```python
from build123d import *

# Parameters (mm, degrees)
F0_W      = 167.5
F0_H      = 92
F1_DEPTH  = 5.5
F2_W      = 137.5
F2_H      = 92
F3_DEPTH  = 49.7
F4_R      = 10
F5_R      = 2.54
F6_R      = 3.3
F6_R_2    = 3
F7_DEPTH  = 5.5
F10_DEPTH = 5.5
F11_R     = 5
F12_R     = 11.129920483
F12_R_2   = 9.5443004054
F13_DEPTH = 10


# Not quite as in the source:
# - a feature names something its author has since deleted; it is built from what else it names


with BuildPart() as f1:
    # F0 (on Top) → F1 (new body)
    with BuildSketch(Plane.XY):
        Rectangle(F0_W, F0_H)
    extrude(amount=F1_DEPTH)

    # F2 (on Top) → F3 (join)
    with BuildSketch(Plane.XY):
        Rectangle(F2_W, F2_H)
    extrude(amount=F3_DEPTH)

    # F4
    f4_edges = [f1.edges().sort_by_distance(p)[0] for p in [
        (-83.75, -46, 2.75),
        (83.75, -46, 2.75),
        (83.75, 46, 2.75),
        (-83.75, 46, 2.75),
        (-68.75, 46, 27.6),
        (-68.75, -46, 27.6),
        (68.75, 46, 27.6),
        (68.75, -46, 27.6),
    ]]
    fillet(f4_edges, radius=F4_R)

    # F5
    f5_edges = [f1.edges().sort_by_distance(p)[0] for p in [
        (0, -46, 49.7),
        (0, 46, 49.7),
        (65.821068, -43.071068, 49.7),
        (68.75, 0, 49.7),
        (65.821068, 43.071068, 49.7),
        (-65.821068, -43.071068, 49.7),
        (-68.75, 0, 49.7),
        (-65.821068, 43.071068, 49.7),
    ]]
    fillet(f5_edges, radius=F5_R)

    # F6 (on face) → F7 (cut)
    with BuildSketch(Plane.XY.offset(5.5)):
        with Locations((-76.25, 22.5)):
            Circle(F6_R)
        with Locations((-76.25, -22.5)):
            Circle(F6_R)
        with Locations((76.25, -22.5)):
            Circle(F6_R)
        with Locations((76.25, 22.5)):
            Circle(F6_R)
        with Locations((76.25, 37.4)):
            Circle(F6_R_2)
        with Locations((76.25, -37.4)):
            Circle(F6_R_2)
    extrude(amount=-F7_DEPTH, mode=Mode.SUBTRACT)

    # F8 (on face) + F9 (on face) → F10 (cut)
    with BuildSketch(Plane.XY.offset(5.5)):
        with BuildLine():
            ThreePointArc((-83.75, -15), (-73.1433982822, -10.6066017178), (-68.75, 0))
            ThreePointArc((-68.75, 0), (-73.1433982822, 10.6066017178), (-83.75, 15))
            Line((-83.75, 15), (-83.75, -15))
        make_face()
    with BuildSketch(Plane.XY.offset(5.5)):
        with BuildLine():
            Line((83.75, -15), (83.75, 15))
            ThreePointArc((83.75, 15), (73.1433983426, 10.6066017782), (68.75, 1.709e-07))
            ThreePointArc((68.75, 1.709e-07), (73.1433982218, -10.6066016574), (83.75, -15))
        make_face()
    extrude(amount=-F10_DEPTH, mode=Mode.SUBTRACT)

    # F11
    f11_edges = [f1.edges().sort_by_distance(p)[0] for p in [
        (83.75, -15, 2.75),
        (-83.75, -15, 2.75),
        (-83.75, 15, 2.75),
        (83.75, 15, 2.75),
    ]]
    fillet(f11_edges, radius=F11_R)

    # F12 (on face) → F13 (join)
    with BuildSketch(Plane.XY.offset(49.7)):
        with Locations((50.4262000322, -21.045640111)):
            Circle(F12_R)
        with Locations((46.4671105146, 16.4614468813)):
            Circle(F12_R_2)
    extrude(amount=F13_DEPTH)


solid = f1.part
```
Geometry check sheet. Reference: the model listing, model coordinates, mm. A direction names the side the tool comes from. Coordinates: 2 decimals unless noted, no trailing zeros. Order: outer loops, then holes, each group sorted by start corner. A loop starts at its lowest first (then second) coordinate and runs counter-clockwise, first axis right, second up. Notation, with made-up numbers: M 48,-32.5 L 94,-32.5 A25 cw 94,2.5 Z; hole C -3,23 d8. An arc over 180 degrees is marked long. Answer as a JSON object with one key per item and string values.
Q1. Cross-section at A-A on x = -76.25. Record the cut outline in (y, z), and give its area (3 significant figures).
Results are:
{"outline": "M -45.68,0 L -25.8,0 L -25.8,5.5 L -45.68,5.5 Z; M -19.2,0 L -12.99,0 L -12.99,5.5 L -19.2,5.5 Z; M 12.99,0 L 19.2,0 L 19.2,5.5 L 12.99,5.5 Z; M 25.8,0 L 45.68,0 L 45.68,5.5 L 25.8,5.5 Z", "area": "287 mm²"}
Q2. Cross-section at B-B on z = 20.5. Record the cut outline in (x, y), and give its area (3 significant figures).
Results are:
{"outline": "M -68.75,-36 A10 ccw -58.75,-46 L 58.75,-46 A10 ccw 68.75,-36 L 68.75,36 A10 ccw 58.75,46 L -58.75,46 A10 ccw -68.75,36 Z", "area": "12,600 mm²"}
Q3. Tool access check on faces 4 (the cylindrical face through (-82.7, 16.3, 2.7)), 5 (the cylindrical face through (82.7, 16.3, 2.7)), 6 (the cylindrical face through (55.6, -30.9, 54.6)), 7 (the cylindrical face through (65.74, 43.15, 26.62)). Record the directions out of +Z, -Z, +X, -X, +Y, -Y that give a thin tool (end or side, any length) a straight path to the whole face; none if there is none.
Results are:
{"face 4": "+Z, -Z, -X", "face 5": "+Z, -Z, +X", "face 6": "+Z", "face 7": "+Z, +X, +Y"}
Q4. Scan lines: line 1 (Y direction, x = 76, z = 1); line 2 (Y direction, x = -76, z = 1); line 3 (Z direction, x = -45.5, y = -13). Record each from-to range of solid material in increasing order.
Results are:
{"line 1": "y = -45.74 to -40.39, -34.41 to -25.79, -19.21 to -12.84, 12.84 to 19.21, 25.79 to 34.41, 40.39 to 45.74", "line 2": "y = -45.74 to -25.79, -19.21 to -12.84, 12.84 to 19.21, 25.79 to 45.74", "line 3": "z = 0 to 49.7"}
Q5. Cross-section at D-D on x = 76.25. Record the cut outline in (y, z).
Results are:
{"outline": "M -45.68,0 L -40.4,0 L -40.4,5.5 L -45.68,5.5 Z; M -34.4,0 L -25.8,0 L -25.8,5.5 L -34.4,5.5 Z; M -19.2,0 L -12.99,0 L -12.99,5.5 L -19.2,5.5 Z; M 12.99,0 L 19.2,0 L 19.2,5.5 L 12.99,5.5 Z; M 25.8,0 L 34.4,0 L 34.4,5.5 L 25.8,5.5 Z; M 40.4,0 L 45.68,0 L 45.68,5.5 L 40.4,5.5 Z"}
Q6. Depth check by flat-ended pin: pin 1 Ø12.5 at (x, y) = (71.5, -34) entering from +Z; pin 2 Ø12.5 at (y, z) = (14, 17) entering from -X; pin 3 Ø8.5 at (x, y) = (76.25, 22.5) entering from +Z. Enter the tip coordinate at first touch or a pass-through.
Results are:
{"pin 1": "stops at z = 49.7", "pin 2": "stops at x = -68.75", "pin 3": "stops at z = 5.5"}
Q7. Cross-section at C-C on y = 22.5. Record the cut outline in (x, z).
Results are:
{"outline": "M -83.75,0 L -79.55,0 L -79.55,5.5 L -83.75,5.5 Z; M -72.95,0 L 72.95,0 L 72.95,5.5 L 68.75,5.5 L 68.75,47.16 A2.54 ccw 66.21,49.7 L 53.86,49.7 L 53.86,59.7 L 39.08,59.7 L 39.08,49.7 L -66.21,49.7 A2.54 ccw -68.75,47.16 L -68.75,5.5 L -72.95,5.5 Z; M 79.55,0 L 83.75,0 L 83.75,5.5 L 79.55,5.5 Z"}
Q8. Release check for a two-part mould opening along Y. For faces 1 (the cylindrical face through (-65.74, -43.15, 26.62)), 2 (the cylindrical face through (55.57, 19.33, 54.63)), 3 (the flat face through (-77, 28, 5.5)) record: released by +Y, released by -Y, zero draft, split by the parting line, or undercut.
Results are:
{"face 1": "released by -Y", "face 2": "undercut", "face 3": "zero draft"}
